Geometry: final body of the model. Coordinates: model frame, mm. A direction names the side the tool comes from. Round coordinates to 2 decimals unless told otherwise and drop trailing zeros. Write each loop counter-clockwise with the first axis right and the second up, starting at its lowest first coordinate (ties: lowest second). Pieces come first, ordered by that corner, then holes.
from build123d import *

# Parameters (mm, degrees)
EXTRUDE_1_DEPTH                = 20
SKETCH_2_W                     = 30
SKETCH_2_H                     = 40
CUT_EXTRUDE_1_DEPTH            = 10
FILLET_1_R                     = 5
FILLET_2_R                     = 1
CUT_EXTRUDE_2_DEPTH            = 37
CUT_EXTRUDE_3_DEPTH            = 190.274932307
CHAMFER_1_SIZE                 = 1
CUT_EXTRUDE_4_DEPTH            = 5
FILLET_3_R                     = 5
PATTERN_LINEAR_7_COUNT         = 2
PATTERN_LINEAR_7_PITCH         = 20
FILLET_3_OF_PATTERN_LINEAR_7_R = 5
SKETCH_7_R                     = 3
CUT_EXTRUDE_5_DEPTH            = 10


# Read off the part's stored shape, not the designer's step: 대칭 복사4
with BuildPart() as part:
    # 스케치1 → 보스-돌출1 (new, symmetric)
    with BuildSketch(Plane.XY):
        Polygon((0, -40), (30, -40), (30, -55), (180, -55), (180, 0), (0, 0), align=None)
    extrude(amount=EXTRUDE_1_DEPTH, both=True)

    # 스케치2 → 컷-돌출1 (cut, symmetric)
    with BuildSketch(Plane.XY):
        with Locations((15, -20)):
            Rectangle(SKETCH_2_W, SKETCH_2_H)
    extrude(amount=CUT_EXTRUDE_1_DEPTH, both=True, mode=Mode.SUBTRACT)

    # 필렛1
    fillet_1_edges = [part.edges().sort_by_distance(p)[0] for p in [
        (180, 0, 0),
    ]]
    fillet(fillet_1_edges, radius=FILLET_1_R)

    # 필렛2
    fillet_2_edges = [part.edges().sort_by_distance(p)[0] for p in [
        (180, -55, 0),
    ]]
    fillet(fillet_2_edges, radius=FILLET_2_R)

    # 스케치3 → 컷-돌출2 (cut)
    with BuildSketch(Plane.ZY):
        with BuildLine():
            Line((-12.990381057, 0), (12.990381057, 0))
            ThreePointArc((12.990381057, 0), (0, -7.5), (-12.990381057, 0))
        make_face()
    extrude(amount=-CUT_EXTRUDE_2_DEPTH, mode=Mode.SUBTRACT)

    # 스케치4 → 컷-돌출3 (cut, through all)
    with BuildSketch(Plane(origin=(180, 0, 0), x_dir=(0, 0, -1), z_dir=(1, 0, 0))):
        with BuildLine():
            Line((-6.614378278, 0), (6.614378278, 0))
            ThreePointArc((6.614378278, 0), (0, -2.5), (-6.614378278, 0))
        make_face()
    extrude(amount=-CUT_EXTRUDE_3_DEPTH, mode=Mode.SUBTRACT)

    # 스케치6 for 컷-로프트1 → 컷-로프트1 section 0
    with BuildSketch(Plane.ZY.offset(-37)):
        with BuildLine():
            Line((-12.990381057, 0), (12.990381057, 0))
            # circular arc as an exact rational Bezier (weights 1, cos(half-angle), 1)
            Bezier((12.990381057, 0), (0, -22.5), (-12.990381057, 0), weights=[1, 0.5, 1])
        make_face()
    # 스케치5 for 컷-로프트1 → 컷-로프트1 section 1
    with BuildSketch(Plane.ZY.offset(-77)):
        with BuildLine():
            Line((-10, 0), (10, 0))
            Bezier((10, 0), (0, -13.333333333), (-10, 0), weights=[1, 0.6, 1])
        make_face()
    loft(mode=Mode.SUBTRACT)

    # 모따기1
    chamfer_1_edges = [part.edges().sort_by_distance(p)[0] for p in [
        (104.5, -55, 20),
        (87.5, 0, 20),
        (180, -29.5, -20),
        (178.535533906, -1.464466094, -20),
        (180, -29.5, 20),
        (178.535533906, -1.464466094, 20),
        (179.707106781, -54.707106781, -20),
        (179.707106781, -54.707106781, 20),
        (87.5, 0, -20),
        (104.5, -55, -20),
    ]]
    chamfer(chamfer_1_edges, length=CHAMFER_1_SIZE)

    # 스케치8 → 컷-돌출4 (cut)
    with BuildSketch(Plane.XY.offset(20)):
        with BuildLine():
            Line((55, -10), (155, -10))
            ThreePointArc((155, -10), (160, -15), (155, -20))
            Line((155, -20), (55, -20))
            ThreePointArc((55, -20), (50, -15), (55, -10))
        make_face()
    cut_extrude_4 = extrude(amount=-CUT_EXTRUDE_4_DEPTH, mode=Mode.SUBTRACT)

    # 필렛3
    fillet_3_edges = [part.edges().sort_by_distance(p)[0] for p in [
        (105, -20, 15),
        (105, -10, 15),
        (50, -15, 15),
        (160, -15, 15),
    ]]
    fillet(fillet_3_edges, radius=FILLET_3_R - 0.0001)  # a hair under: the kernel refuses the full size

    # 선형 패턴7: 컷-돌출4 ×2
    with Locations(*[(0, -i * PATTERN_LINEAR_7_PITCH, 0) for i in range(1, PATTERN_LINEAR_7_COUNT)]):
        add(cut_extrude_4, mode=Mode.SUBTRACT)

    # 필렛3 of 선형 패턴7
    fillet_3_of_pattern_linear_7_edges = [part.edges().sort_by_distance(p)[0] for p in [
        (105, -40, 15),
        (105, -30, 15),
        (50, -35, 15),
        (160, -35, 15),
    ]]
    fillet(fillet_3_of_pattern_linear_7_edges, radius=FILLET_3_OF_PATTERN_LINEAR_7_R - 0.0001)  # a hair under: the kernel refuses the full size

    # 대칭 복사4 outline → 대칭 복사4 (revolve, cut)
    with BuildSketch(Plane(origin=(0, -15, -20), x_dir=(0, 1, 0), z_dir=(0, 0, -1))):
        with BuildLine():
            ThreePointArc((0, 50), (3.535533906, 51.464466094), (5, 55))
            Line((5, 55), (5, 155))
            ThreePointArc((5, 155), (3.535533906, 158.535533906), (0, 160))
            Line((0, 160), (0, 50))
        make_face()
    revolve(axis=Axis((0, -15, -20), (1, 0, 0)), mode=Mode.SUBTRACT)

    # Mirror 4 2 outline → Mirror 4 2 (revolve, cut)
    with BuildSketch(Plane(origin=(0, -35, -20), x_dir=(0, 1, 0), z_dir=(0, 0, -1))):
        with BuildLine():
            ThreePointArc((0, 50), (3.535533906, 51.464466094), (5, 55))
            Line((5, 55), (5, 155))
            ThreePointArc((5, 155), (3.535533906, 158.535533906), (0, 160))
            Line((0, 160), (0, 50))
        make_face()
    revolve(axis=Axis((0, -35, -20), (1, 0, 0)), mode=Mode.SUBTRACT)

    # 스케치7 → 컷-돌출5 (cut)
    with BuildSketch(Plane.XZ.offset(55)):
        with Locations(Location((165, 0, 0), (0, 0, 270))):
            Circle(SKETCH_7_R)
        with Locations(Location((110, 0, 0), (0, 0, 270))):
            Circle(SKETCH_7_R)
    extrude(amount=-CUT_EXTRUDE_5_DEPTH, mode=Mode.SUBTRACT)


solid = part.part
1) Section A-A on x = 165. Output: boundary loops of the cut face in (y, z), plus the area to 3 significant figures.
2) Reachability of faces 1 (the cylindrical face through (106, -15, -15)), 2 (the cylindrical face through (106, -31, 17)), 3 (the flat face through (15, -40, 15)), 4 (the flat face through (77, -3, 0)) from +Z, -Z, +X, -X, +Y, -Y: full face, straight path, thin tool, end or side. Return the list, or none.
3) First-contact query: P1, Ø7, axis at x = 110, z = 0, coming from the -Y side; P2, Ø8, axis at x = 13.5, z = 13, coming from the -Y side; P3, Ø3, axis at x = 111, y = -18, coming from the -Z side; P4, Ø3, axis at x = 110.5, z = 0, coming from the -Y side. Flat tips, straight axial feed; report the tip coordinate or a pass-through.
4) Line query: probe 1 along X at (y, z) = (-53, 0); probe 2 along Z at (x, y) = (165, -52); probe 3 along Z at (x, y) = (14, -13). Output: solid intervals per line, ascending.
5) Draft query along X for faces 5 (the cylindrical face through (104, -19, 17)), 6 (the cylindrical face through (106, -11, 17)), 7 (the cylindrical face through (179.51, -2.84, -0.27)), 8 (the cylindrical face through (128.9, -2.5, -0.1)). Return one class per face: pulls with the +X half, pulls with the -X half, needs draft (parallel to the pull), parting line crosses it, or undercut.
Filled in:
1. outline: (-55, -19) - (-54, -20) - (-1, -20) - (0, -19) - (0, -6.61) arc R10 cw to (0, 6.61) - (0, 19) - (-1, 20) - (-54, 20) - (-55, 19) - (-55, 3) - (-45, 3) - (-45, -3) - (-55, -3) - close
1. area: 2,120 mm2
2. face 1: -Z
2. face 2: +Z
2. face 3: +Z, -Z, -X, -Y
2. face 4: -X, +Y
3. P1: stops at y = -55
3. P2: stops at y = -40
3. P3: stops at z = -17.82
3. P4: stops at y = -45
4. probe 1: x = 30 to 107, 113 to 162, 168 to 180
4. probe 2: z = -20 to -3, 3 to 20
4. probe 3: z = -20 to -10, 10 to 20
5. face 5: undercut
5. face 6: undercut
5. face 7: pulls with the +X half
5. face 8: needs draft
